from build123d import *

# Parameters (mm, degrees)
SKETCH3_R          = 1
CUT_EXTRUDE1_DEPTH = 4
SKETCH5_R          = 1
CUT_EXTRUDE2_DEPTH = 3


with BuildPart() as part:
    # Sketch2 → Revolve2 (revolve)
    with BuildSketch(Plane.XY, mode=Mode.PRIVATE) as revolve2_sk:
        Polygon((0, 0), (0, 22), (1, 22), (1, 18.5), (7.5, 18.5), (11.5, 14.5), (11.5, 4.8), (9.5, 4.8), (9.5, 4.5), (11.5, 4.5), (11.5, 3.5), (11, 3.5), (11, 3), (11.5, 3), (11.5, 2), (9.5, 0), (2, 0), (2, -1.8), (0, -1.8), align=None)
        Polygon((1, 16.5), (1, 10.79), (10.5, 10.79), (10.5, 14.085786438), (7.085786438, 17.5), (2, 17.5), (2, 16.5), align=None, mode=Mode.SUBTRACT)
    revolve(revolve2_sk.sketch.rotate(Axis((0, 0, 0), (0, 1, 0)), 90), axis=Axis((0, 0, 0), (0, 1, 0)))

    # Sketch3 → Cut-Extrude1 (cut)
    with BuildSketch(Plane(origin=(0, 18.5, 0), x_dir=(1, 0, 0), z_dir=(0, 1, 0))):
        with Locations(Location((0, 4.5, 0), (0, 0, 270))):
            Circle(SKETCH3_R)
        with Locations(Location((4.5, 0, 0), (0, 0, 270))):
            Circle(SKETCH3_R)
        with Locations(Location((0, -4.5, 0), (0, 0, 270))):
            Circle(SKETCH3_R)
        with Locations(Location((-4.5, 0, 0), (0, 0, 270))):
            Circle(SKETCH3_R)
        with BuildLine():
            Line((3, 9), (3, 18.27))
            Line((3, 18.27), (-3, 18.27))
            Line((-3, 18.27), (-3, 9))
            ThreePointArc((-3, 9), (0, 6), (3, 9))
        make_face()
        with BuildLine():
            Line((9, -3), (18.27, -3))
            Line((18.27, -3), (18.27, 3))
            Line((18.27, 3), (9, 3))
            ThreePointArc((9, 3), (6, 0), (9, -3))
        make_face()
        with BuildLine():
            Line((-3, -9), (-3, -18.27))
            Line((-3, -18.27), (3, -18.27))
            Line((3, -18.27), (3, -9))
            ThreePointArc((3, -9), (0, -6), (-3, -9))
        make_face()
        with BuildLine():
            Line((-9, 3), (-18.27, 3))
            Line((-18.27, 3), (-18.27, -3))
            Line((-18.27, -3), (-9, -3))
            ThreePointArc((-9, -3), (-6, 0), (-9, 3))
        make_face()
    extrude(amount=-CUT_EXTRUDE1_DEPTH, mode=Mode.SUBTRACT)

    # Sketch5 → Cut-Extrude2 (cut)
    with BuildSketch(Plane.XZ):
        with Locations(Location((0, 6, 0), (0, 0, 270))):
            Circle(SKETCH5_R)
        with Locations(Location((6, 0, 0), (0, 0, 270))):
            Circle(SKETCH5_R)
        with Locations(Location((0, -6, 0), (0, 0, 270))):
            Circle(SKETCH5_R)
        with Locations(Location((-6, 0, 0), (0, 0, 270))):
            Circle(SKETCH5_R)
    extrude(amount=-CUT_EXTRUDE2_DEPTH, mode=Mode.SUBTRACT)


solid = part.part
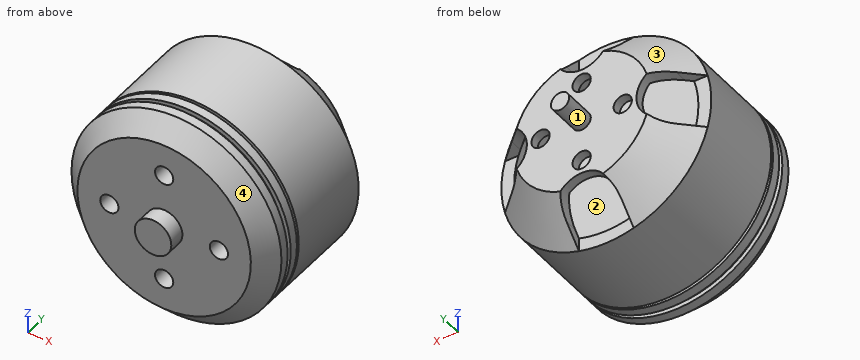
Work out the finished part from the listing and answer in its coordinate system (mm). Face numbers are marked on the shaded views. Give positions to 0.01 mm unless a question says otherwise; leave off trailing zeros. Write each loop counter-clockwise with the first axis right and the second up, starting at its lowest first coordinate (ties: lowest second). Pieces come first, ordered by that corner, then holes. Notation, with made-up numbers: (-40, 88) - (4, 88) arc R10 cw to (4, 92) - close; hole circle Ø4 at (1, 72.25). An arc over 180 degrees is marked (long way). One line per item, written item: value. Start each with the question number.
1. Find section B-B (y = 19.25). Write down the section's boundary in (x, z), then the cut area to 3 significant figures.
2. Consider probe 1 along X at (y, z) = (12.8, 0); probe 2 along Y at (x, z) = (-1.5, -5); probe 3 along Y at (x, z) = (6, 7.75). Determine where each line is inside the solid, lowest interval first.
3. Find section C-C (x = 0). State how many separate pieces and enclosed holes the cut face has, then the cut area to 3 significant figures.
4. Given pin 1 (2 mm diameter, centred on x = -0.5, z = -6.5, fed in from -Y); pin 2 (4 mm diameter, centred on x = -3.5, y = 2.5, fed in from -Z); pin 3 (7 mm diameter, centred on x = -3, z = 4.5, fed in from +Y); pin 4 (6 mm diameter, centred on y = 14, z = 0.5, fed in from +X), each flat-ended and moving along its own axis, determine where each tip first touches the part or whether it passes through.
5. Find section A-A (y = 12). Write down the section's boundary in (x, z), then the cut area to 3 significant figures.
6. For a pull along Y with two mould halves and no side action, classify the marked faces 1, 2, 3 and 4 as +Y half, -Y half, draft (parallel to the pull), parting line (faces both ways), or undercut.
Geometry results:
1. outline: circle Ø2 at (0, 0)
1. area: 3.14 mm2
2. probe 1: -11.5 to -10.5, -1 to 1, 10.5 to 11.5
2. probe 2: 0 to 10.79, 17.5 to 18.5
2. probe 3: 0.3 to 4.5, 4.8 to 10.79, 14.78 to 16.2
3. separate pieces: 3
3. enclosed holes: 0
3. area: 276 mm2
4. pin 1: y = 0
4. pin 2: z = -11.4
4. pin 3: y = 18.5
4. pin 4: x = 11.5
5. outline: circle Ø23 at (0, 0); circle Ø2 at (0, 0); hole circle Ø21 at (0, 0)
5. area: 72.3 mm2
6. face 1: draft
6. face 2: undercut
6. face 3: +Y half
6. face 4: -Y half
